Can you work these out from the model? Positions are in its coordinate system, mm. Face numbers are marked on the shaded views. Give positions to 0.01 mm unless a question says otherwise; leave off trailing zeros. Order: outer loops, then holes, each group sorted by start corner. A loop starts at its lowest first (then second) coordinate and runs counter-clockwise, first axis right, second up. Notation, with made-up numbers: (14.25, -10) -> (34.25, -10) arc R36 cw to (34.25, 26) -> close; hole circle Ø9 at (5.5, -24.75). An arc over 180 degrees is marked (long way). Answer as CSV lines item,"result".
```python
from build123d import *

# Parameters (mm, degrees)
SKETCH1_W           = 16.3
SKETCH1_H           = 16.3
BOSS_EXTRUDE1_DEPTH = 12.3
SKETCH2_R           = 3
CUT_EXTRUDE1_DEPTH  = 12.3


with BuildPart() as part:
    # Sketch1 → Boss-Extrude1 (new body)
    with BuildSketch(Plane(origin=(0, 0, 0), x_dir=(1, 0, 0), z_dir=(0, 1, 0))):
        Rectangle(SKETCH1_W, SKETCH1_H)
    extrude(amount=BOSS_EXTRUDE1_DEPTH)

    # Sketch2 → Cut-Extrude1 (cut)
    with BuildSketch(Plane(origin=(0, 0, 0), x_dir=(1, 0, 0), z_dir=(0, 1, 0))):
        with Locations(Location((3.65, 0, 0), (0, 0, 90))):
            Circle(SKETCH2_R)
    extrude(amount=CUT_EXTRUDE1_DEPTH, mode=Mode.SUBTRACT)


solid = part.part
```
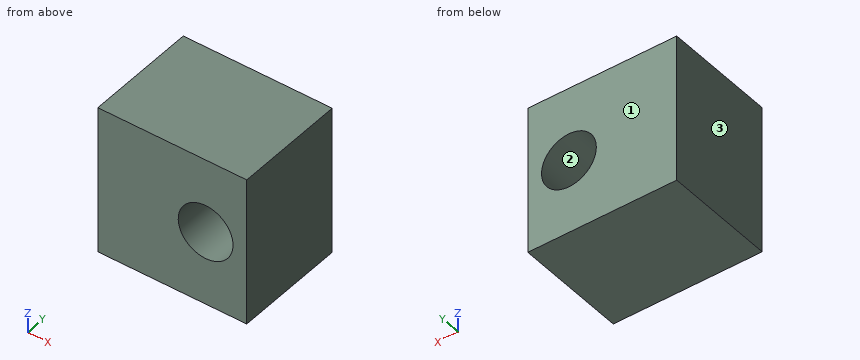
Item 1: Imagine slicing it at B-B, the plane x = 3.65. Please give me the cut outline in (y, z), then the cut area to 3 significant figures.
Numbers:
outline,"(0, -8.15) -> (12.3, -8.15) -> (12.3, -3) -> (0, -3) -> close; (0, 3) -> (12.3, 3) -> (12.3, 8.15) -> (0, 8.15) -> close"
area,"127 mm²"
Item 2: Imagine slicing it at C-C, the plane y = 7. Please give me the cut outline in (x, z), then the cut area to 3 significant figures.
Numbers:
outline,"(-8.15, -8.15) -> (8.15, -8.15) -> (8.15, 8.15) -> (-8.15, 8.15) -> close; hole circle Ø6 at (3.65, 0)"
area,"237 mm²"
Item 3: We'd pull the mould along X, two halves only. Please class the marked faces 1, 2 and 3: released by +X, released by -X, zero draft, split by the parting line, or undercut.
Numbers:
face 1,"zero draft"
face 2,"undercut"
face 3,"released by -X"
Item 4: Imagine slicing it at A-A, the plane z = 0. Please give me the cut outline in (x, y), then the cut area to 3 significant figures.
Numbers:
outline,"(-8.15, 0) -> (0.65, 0) -> (0.65, 12.3) -> (-8.15, 12.3) -> close; (6.65, 0) -> (8.15, 0) -> (8.15, 12.3) -> (6.65, 12.3) -> close"
area,"127 mm²"
Item 5: Please list where these lines run through material, in increasing order: line 1 along X through (y, z) = (7.5, 0); line 2 along Z through (x, y) = (3.5, 2.5); line 3 along Z through (x, y) = (3, 9.25).
Numbers:
line 1,"x = -8.15 to 0.65, 6.65 to 8.15"
line 2,"z = -8.15 to -3, 3 to 8.15"
line 3,"z = -8.15 to -2.93, 2.93 to 8.15"
